Read the model definition and answer for the solid it produces. Units are mm, in the model's axes. Face numbers are marked on the shaded views. A direction names the side the tool comes from. Coordinates: 2 decimals unless noted, no trailing zeros. Write each loop counter-clockwise with the first axis right and the second up, starting at its lowest first coordinate (ties: lowest second). Pieces come first, ordered by that corner, then holes.
Item 1: Section B-B (z = 18.25) is taken. Give the vertices of the cut face in (x, y), then the cut area to 3 significant figures.
Item 2: Section D-D (y = -20.5) is taken. Give the vertices of the cut face in (x, z), then the cut area to 3 significant figures.
Item 3: Section C-C (x = -5.5) is taken. Give the vertices of the cut face in (y, z).
Item 4: Each of these flat-tipped pins is pushed along its axis until it touches: P1, Ø8, axis at y = -24.5, z = 13.5, coming from the -X side; P2, Ø6, axis at y = -16, z = 11, coming from the -X side; P3, Ø8, axis at y = -55.5, z = 12.5, coming from the -X side. Where does it stop, or does it pass through?
Item 5: Straight lines are drawn through the part: probe 1 along X at (y, z) = (-10.5, 8); probe 2 along X at (y, z) = (-28, 8); probe 3 along Y at (x, z) = (-54.5, 6.5). For each, find the intervals that lie inside material, in ascending order.
Item 6: Determine the mould class of the marked faces 4, 5 and 6 for opening direction X: released by +X, released by -X, zero draft, split by the parting line, or undercut.
Item 7: Section A-A (y = -51) is taken. Give the vertices of the cut face in (x, z), then the cut area to 3 significant figures.
Item 8: A tool of negligible diameter and unlimited length cuts with its end or side. For the marked faces 1, 2 and 3, from which of +Z, -Z, +X, -X, +Y, -Y can it reach the whole face along a straight path? Write none if from no direction.
from build123d import *

# Parameters (mm, degrees)
F1_DEPTH = 20


with BuildPart() as f1:
    # F0 (on Top) → F1 (new body)
    with BuildSketch(Plane.XY):
        Polygon((23.470087, -5), (23.470087, 0), (-71.529913, 0), (-71.529913, 5), (-76.529913, 5), (-76.529913, 0), (-76.529913, -5), (-67.359267, -5), (-28.059433, -5), (-23.059433, -5), (14.299441, -5), align=None)
        Polygon((23.470087, -64.074456), (23.470087, -5), (14.299441, -5), (14.299441, -58.109964), align=None)
        Polygon((14.299441, -64.074456), (23.470087, -64.074456), (14.299441, -58.109964), align=None)
        Polygon((14.299441, -64.074456), (14.299441, -58.109964), (-23.059433, -33.812146), (-28.059433, -30.560198), (-67.359267, -5), (-76.529913, -5), align=None)
        Polygon((-23.059433, -33.812146), (-23.059433, -5), (-28.059433, -5), (-28.059433, -30.560198), align=None)
    extrude(amount=F1_DEPTH)


solid = f1.part
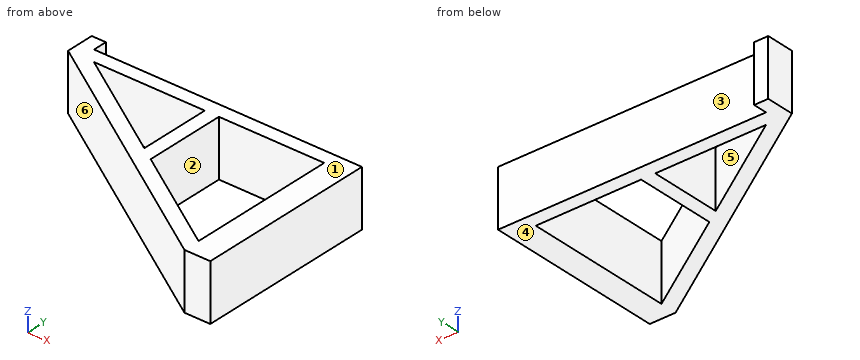
Established:
1. outline: (-76.53, -5) - (14.3, -64.07) - (23.47, -64.07) - (23.47, 0) - (-71.53, 0) - (-71.53, 5) - (-76.53, 5) - close; hole (-67.36, -5) - (-28.06, -30.56) - (-28.06, -5) - close; hole (-23.06, -33.81) - (14.3, -58.11) - (14.3, -5) - (-23.06, -5) - close
1. area: 1,720 mm2
2. outline: (-52.7, 0) - (-43.53, 0) - (-43.53, 20) - (-52.7, 20) - close; (-28.06, 0) - (-23.06, 0) - (-23.06, 20) - (-28.06, 20) - close; (14.3, 0) - (23.47, 0) - (23.47, 20) - (14.3, 20) - close
2. area: 467 mm2
3. outline: (-51.2, 0) - (-45.23, 0) - (-45.23, 20) - (-51.2, 20) - close; (-5, 0) - (0, 0) - (0, 20) - (-5, 20) - close
4. P1: stops at x = -52.7
4. P2: stops at x = -64.23
4. P3: stops at x = -5.03
5. probe 1: x = -68.07 to -58.9, -28.06 to -23.06, 14.3 to 23.47
5. probe 2: x = -41.17 to -32, -28.06 to -23.06, 14.3 to 23.47
5. probe 3: y = -19.33 to -13.36, -5 to 0
6. face 4: zero draft
6. face 5: undercut
6. face 6: released by -X
7. outline: (-5.8, 0) - (3.37, 0) - (3.37, 20) - (-5.8, 20) - close; (14.3, 0) - (23.47, 0) - (23.47, 20) - (14.3, 20) - close
7. area: 367 mm2
8. face 1: +Z, +X, -X, +Y, -Y
8. face 2: +Z, -Z
8. face 3: +Z, -Z, +X, +Y
